The model under review builds one solid part; all positions refer to its coordinate system, in mm. A direction names the side the tool comes from. Coordinates: 2 decimals unless noted, no trailing zeros. Order: outer loops, then holes, each group sorted by start corner. A loop starts at its lowest first (then second) coordinate and runs counter-clockwise, first axis right, second up. Notation, with made-up numbers: (24.25, 25.5) - (59.25, 25.5) arc R26 ccw to (59.25, 61.5) - close; hole circle Ø1 at (-36.5, -25). An arc over 180 degrees is marked (long way). Answer in a Markdown table with one row per item.
```python
from build123d import *

# Parameters (mm, degrees)
F0_R     = 0.9278723563
F1_DEPTH = 12.7
F4_DEPTH = 7.62
F5_R     = 5.8500473035
F6_DEPTH = 1.27


with BuildPart() as f1:
    # F0 (on Top) → F1 (new body, symmetric)
    with BuildSketch(Plane.XY):
        Circle(F0_R)
    extrude(amount=F1_DEPTH, both=True)

    # F2 (on Front) → F3 (revolve)
    with BuildSketch(Plane.XZ):
        Polygon((0, -15.8198643476), (0, -12.7), (-2.3196195252, -12.7), align=None)
    revolve(axis=Axis((0, 0, -14.2599321738), (0, 0, 1)))

    # F4 (cut): a face of the model
    f4_faces = [f1.faces().sort_by_distance(p)[0] for p in [
        (0, 0, 12.7),
    ]]
    extrude(f4_faces, amount=-F4_DEPTH, mode=Mode.SUBTRACT)

    # F5 (on Top) → F6 (join)
    with BuildSketch(Plane.XY):
        Circle(F5_R)
    extrude(amount=F6_DEPTH)


solid = f1.part
```
Item 1: Mouldability with a two-part tool opening along Z and no side actions: class faces 3 (the face through (0.5, 1, -12.7)), 4 (the face through (1.2, 0.1, 1.27)), 5 (the face through (-1.27, -5.71, 0.63)), 6 (the face through (-0.201, -0.906, -6.261)) as +Z half, -Z half, draft (parallel to the pull), parting line (faces both ways), or undercut.
Check values:
| item | result |
|---|---|
| face 3 | undercut |
| face 4 | +Z half |
| face 5 | draft |
| face 6 | undercut |
Item 2: We need section B-B, the plane y = 4. Write out the cut boundary in (x, z), then the cut area to 3 significant figures.
Check values:
| item | result |
|---|---|
| outline | (-4.27, 0) - (4.27, 0) - (4.27, 1.27) - (-4.27, 1.27) - close |
| area | 10.8 mm^2 |
Item 3: To check wall thickness, follow line 1 (Z direction, x = -2, y = -2); line 2 (Y direction, x = 0, z = -11.75); line 3 (X direction, y = -4.25, z = 1). State the ranges of each line that lie inside material, in increasing order. Write a range as from..to.
Check values:
| item | result |
|---|---|
| line 1 | 0..1.27 |
| line 2 | -0.93..0.93 |
| line 3 | -4.02..4.02 |
Item 4: We need section A-A, the plane z = 2.75. Write out the cut boundary in (x, y), then the cut area to 3 significant figures.
Check values:
| item | result |
|---|---|
| outline | circle Ø1.86 at (0, 0) |
| area | 2.70 mm^2 |
Item 5: Tool access review of faces 1 (the face through (-0.201, -0.906, 3.202)), 2 (the face through (0.1, 0.6, -15)): name each direction out of +Z, -Z, +X, -X, +Y, -Y from which nothing blocks a thin tool from reaching the whole face with its end or side.
Check values:
| item | result |
|---|---|
| face 1 | +Z |
| face 2 | -Z |
Item 6: We need section C-C, the plane x = -3. Write out the cut boundary in (y, z).
Check values:
| item | result |
|---|---|
| outline | (-5.02, 0) - (5.02, 0) - (5.02, 1.27) - (-5.02, 1.27) - close |
Item 7: Clearance check with flat-ended pins moving along their axes: pin 1 Ø3 at (x, z) = (3, 3) entering from +Y; pin 2 Ø1 at (x, y) = (2.5, 2) entering from +Z; pin 3 Ø4 at (x, y) = (-2, -4) entering from -Z; pin 4 Ø1.5 at (x, z) = (0, -8.5) entering from +Y. State where each tip first meets the part, or that it passes through.
Check values:
| item | result |
|---|---|
| pin 1 | through |
| pin 2 | z = 1.27 |
| pin 3 | z = 0 |
| pin 4 | y = 0.93 |
